from build123d import *

# Parameters (mm, degrees)
F1_DEPTH = 6.35
F2_R     = 15.316097
F3_DEPTH = 6.35
F2_R_2   = 17.868779
F4_DEPTH = 2.54
F2_R_3   = 1.5875
F5_DEPTH = 6.35
F2_R_4   = 2.7305
F2_R_5   = 2.726201
F6_DEPTH = 3.048


with BuildPart() as f1:
    # F0 (on Front) → F1 (new body)
    with BuildSketch(Plane.XZ):
        with BuildLine():
            ThreePointArc((73.025, 60.325), (69.305256, 69.305256), (60.325, 73.025))
            Line((60.325, 73.025), (-60.325, 73.025))
            ThreePointArc((-60.325, 73.025), (-69.305256, 69.305256), (-73.025, 60.325))
            Line((-73.025, 60.325), (-73.025, -60.325))
            ThreePointArc((-73.025, -60.325), (-69.305256, -69.305256), (-60.325, -73.025))
            Line((-60.325, -73.025), (60.325, -73.025))
            ThreePointArc((60.325, -73.025), (69.305256, -69.305256), (73.025, -60.325))
            Line((73.025, -60.325), (73.025, 60.325))
        make_face()
    extrude(amount=F1_DEPTH)

    # F2 (on face) → F3 (cut)
    with BuildSketch(Plane.XZ.offset(6.35)):
        Circle(F2_R)
    extrude(amount=-F3_DEPTH, mode=Mode.SUBTRACT)

    # F2 (on face) → F4 (cut)
    with BuildSketch(Plane.XZ.offset(6.35)):
        Circle(F2_R_2)
        Circle(F2_R, mode=Mode.SUBTRACT)
    extrude(amount=-F4_DEPTH, mode=Mode.SUBTRACT)

    # F2 (on face) → F5 (cut)
    with BuildSketch(Plane.XZ.offset(6.35)):
        with Locations((30.1625, 30.1625)):
            Circle(F2_R_3)
        with Locations((30.1625, -30.1625)):
            Circle(F2_R_3)
        with Locations((-30.1625, 30.1625)):
            Circle(F2_R_3)
        with Locations((-30.1625, -30.1625)):
            Circle(F2_R_3)
    extrude(amount=-F5_DEPTH, mode=Mode.SUBTRACT)

    # F2 (on face) → F6 (cut)
    with BuildSketch(Plane.XZ.offset(6.35)):
        with Locations((-30.1625, -30.1625)):
            Circle(F2_R_4)
        with Locations((-30.1625, -30.1625)):
            Circle(F2_R_3, mode=Mode.SUBTRACT)
        with Locations((30.1625, -30.1625)):
            Circle(F2_R_4)
        with Locations((30.1625, -30.1625)):
            Circle(F2_R_3, mode=Mode.SUBTRACT)
        with Locations((30.1625, 30.1625)):
            Circle(F2_R_4)
        with Locations((30.1625, 30.1625)):
            Circle(F2_R_3, mode=Mode.SUBTRACT)
        with Locations((-30.1625, 30.1625)):
            Circle(F2_R_5)
        with Locations((-30.1625, 30.1625)):
            Circle(F2_R_3, mode=Mode.SUBTRACT)
    extrude(amount=-F6_DEPTH, mode=Mode.SUBTRACT)


solid = f1.part
Geometry: final body of the model. Coordinates: model frame, mm. A direction names the side the tool comes from. Round coordinates to 2 decimals unless told otherwise and drop trailing zeros. Order: outer loops, then holes, each group sorted by start corner. A loop starts at its lowest first (then second) coordinate and runs counter-clockwise, first axis right, second up. Notation, with made-up numbers: (55.25, 24) -> (71.25, 24) arc R21 cw to (71.25, 62) -> close; hole circle Ø5 at (60, 16). An arc over 180 degrees is marked (long way). Put each result on its own line as item: value. Start each with the question number.
Q1. Pull-direction query (Z, two-part tool) for faces 1 (the flat face through (-1, -3, -73.025)), 2 (the flat face through (32, -3.302, -30)), 3 (the flat face through (73.025, -3, -1)); classes: +Z half, -Z half, draft (parallel to the pull), parting line (faces both ways), or undercut.
Q2. Section B-B on z = 0. Return the cut outline in (x, y) (3 decimals).
Q3. First-contact query: pin 1 (10.5 mm diameter, centred on x = 4.5, z = 6.5, fed in from -Y); pin 2 (1.6 mm diameter, centred on x = 31.5, z = -29, fed in from -Y); pin 3 (4 mm diameter, centred on x = -30.16, z = -30.16, fed in from +Y). Flat tips, straight axial feed; report the tip coordinate or a pass-through.
Q4. Section C-C on y = -2. Give the number of separate pieces and of enclosed holes in the cut face, and give its area (3 significant figures).
Q5. Line query: probe 1 along Z at (x, y) = (-28, -4.25) (3 decimals); probe 2 along X at (y, z) = (-4, 61); probe 3 along X at (y, z) = (-6, -11) (3 decimals). Output: solid intervals per line, ascending.
Q6. Reachability of faces 4 (the flat face through (1, -3, 73.025)), 5 (the cylindrical face through (31.422, -4.847, -32.585)) from +Z, -Z, +X, -X, +Y, -Y: full face, straight path, thin tool, end or side. Return the list, or none.
Q7. Section A-A on x = 0. Return the cut outline in (y, z) (3 decimals), and give its area (3 significant figures).
Ans:
1. face 1: -Z half
1. face 2: undercut
1. face 3: draft
2. outline: (-73.025, -6.35) -> (-17.869, -6.35) -> (-17.869, -3.81) -> (-15.316, -3.81) -> (-15.316, 0) -> (-73.025, 0) -> close; (15.316, -3.81) -> (17.869, -3.81) -> (17.869, -6.35) -> (73.025, -6.35) -> (73.025, 0) -> (15.316, 0) -> close
3. pin 1: passes through
3. pin 2: stops at y = -3.3
3. pin 3: stops at y = 0
4. separate pieces: 1
4. enclosed holes: 5
4. area: 20,400 mm2
5. probe 1: z = -73.025 to -31.83, -28.495 to 28.502, 31.823 to 73.025
5. probe 2: x = -73.01 to 73.01
5. probe 3: x = -73.025 to -14.082, 14.082 to 73.025
6. face 4: +Z, +X, -X, +Y, -Y
6. face 5: -Y
7. outline: (-6.35, -73.025) -> (0, -73.025) -> (0, -15.316) -> (-3.81, -15.316) -> (-3.81, -17.869) -> (-6.35, -17.869) -> close; (-6.35, 17.869) -> (-3.81, 17.869) -> (-3.81, 15.316) -> (0, 15.316) -> (0, 73.025) -> (-6.35, 73.025) -> close
7. area: 720 mm2
